Check sheet for the modelled part. Datum: model origin and axes. Units: mm. A direction names the side the tool comes from. Round coordinates to 2 decimals unless told otherwise and drop trailing zeros. Write each loop counter-clockwise with the first axis right and the second up, starting at its lowest first coordinate (ties: lowest second). Pieces come first, ordered by that corner, then holes. Notation, with made-up numbers: M -13.75,32 L 5.25,32 A18 cw 5.25,44 Z; hole C 58.5,-32 d9. An arc over 180 degrees is marked long. One line per item, written item: value.
from build123d import *

# Parameters (mm, degrees)
BOSS_EXTRUDE1_DEPTH = 3.175
SKETCH3_R           = 1.65
CUT_EXTRUDE1_DEPTH  = 3.175


with BuildPart() as part:
    # Sketch2 → Boss-Extrude1 (new body)
    with BuildSketch(Plane(origin=(0, 0, 0), x_dir=(1, 0, 0), z_dir=(0, 1, 0))):
        with BuildLine():
            Line((-145.521414695, 0.997059393), (-107.921414695, 0.997059393))
            ThreePointArc((-107.921414695, 0.997059393), (-92.921414695, -14.002940607), (-107.921414695, -29.002940607))
            Line((-107.921414695, -29.002940607), (-145.521414695, -29.002940607))
            ThreePointArc((-145.521414695, -29.002940607), (-160.521414695, -14.002940607), (-145.521414695, 0.997059393))
        make_face()
        Polygon((-149.500688753, -12.502940607), (-147.479962811, -9.002940607), (-149.500688753, -5.502940607), (-153.542140637, -5.502940607), (-155.562866579, -9.002940607), (-153.542140637, -12.502940607), align=None, mode=Mode.SUBTRACT)
        Polygon((-153.542140637, -15.502940607), (-149.500688753, -15.502940607), (-147.479962811, -19.002940607), (-149.500688753, -22.502940607), (-153.542140637, -22.502940607), (-155.562866579, -19.002940607), align=None, mode=Mode.SUBTRACT)
        Polygon((-103.942140637, -15.502940607), (-105.962866579, -19.002940607), (-103.942140637, -22.502940607), (-99.900688753, -22.502940607), (-97.879962811, -19.002940607), (-99.900688753, -15.502940607), align=None, mode=Mode.SUBTRACT)
        Polygon((-99.900688753, -12.502940607), (-103.942140637, -12.502940607), (-105.962866579, -9.002940607), (-103.942140637, -5.502940607), (-99.900688753, -5.502940607), (-97.879962811, -9.002940607), align=None, mode=Mode.SUBTRACT)
    extrude(amount=BOSS_EXTRUDE1_DEPTH)

    # Sketch3 → Cut-Extrude1 (cut)
    with BuildSketch(Plane.XZ):
        with Locations(Location((-136.722782871, 13.998131439, 0), (0, 0, 270))):
            Circle(SKETCH3_R)
    extrude(amount=-CUT_EXTRUDE1_DEPTH, mode=Mode.SUBTRACT)


solid = part.part
Q1. Sectioned sample at B-B on y = 2.1. State how many separate pieces and enclosed holes the cut face has, and give its area (3 significant figures).
Completed:
separate pieces: 1
enclosed holes: 5
area: 1,660 mm^2
Q2. Sectioned sample at A-A on z = 6.5. Enter the section's corners in (x, y) (3 decimals).
Completed:
outline: M -158.51,0 L -154.118,0 L -154.118,3.175 L -158.51,3.175 Z; M -148.925,0 L -104.518,0 L -104.518,3.175 L -148.925,3.175 Z; M -99.325,0 L -94.933,0 L -94.933,3.175 L -99.325,3.175 Z
Q3. Depth check by flat-ended pin: P1, Ø1.5, axis at x = -152.5, y = 1.5, coming from the -Z side; P2, Ø1, axis at x = -104.5, y = 2, coming from the -Z side; P3, Ø1.6, axis at x = -101, y = 1.5, coming from the -Z side. Enter the tip coordinate at first touch or a pass-through.
Completed:
P1: z = 0.36
P2: z = -0.71
P3: z = 0.31
Q4. Draft check along X on faces 3 (the cylindrical face through (-160.518, 1.565, 14.333)), 4 (the flat face through (-152, 2, 12.503)), 5 (the flat face through (-104.94, 1.57, 17.23)), 6 (the flat face through (-126, 0, 14)). Enter one of: pulls with the +X half, pulls with the -X half, needs draft (parallel to the pull), parting line crosses it, or undercut.
Completed:
face 3: pulls with the -X half
face 4: undercut
face 5: undercut
face 6: needs draft
Q5. Sectioned sample at C-C on z = 10. Enter the section's corners in (x, y) (3 decimals).
Completed:
outline: M -159.977,0 L -154.987,0 L -154.987,3.175 L -159.977,3.175 Z; M -148.056,0 L -105.387,0 L -105.387,3.175 L -148.056,3.175 Z; M -98.456,0 L -93.465,0 L -93.465,3.175 L -98.456,3.175 Z
Q6. Scan lines: line 1 (Z direction, x = -152, y = 2.6); line 2 (X direction, y = 1.15, z = 11); line 3 (X direction, y = 2.55, z = 6.5). Record each from-to range of solid material in increasing order. Write a range as [from, to].
Completed:
line 1: [0.47, 5.5], [12.5, 15.5], [22.5, 27.53]
line 2: [-160.22, -154.41], [-148.63, -104.81], [-99.03, -93.23]
line 3: [-158.51, -154.12], [-148.93, -104.52], [-99.33, -94.93]
Q7. Sectioned sample at D-D on z = 26.75. Enter the section's corners in (x, y) (3 decimals).
Completed:
outline: M -153.428,0 L -100.015,0 L -100.015,3.175 L -153.428,3.175 Z
Q8. Access from +Z, -Z, +X, -X, +Y, -Y to the whole of each face (thin tool, end or side, straight path). Record for faces 1 (the flat face through (-126, 2, 29.003)), 2 (the flat face through (-104.967, 1.565, 20.728)).
Completed:
face 1: +Z, +X, -X, +Y, -Y
face 2: +Y, -Y
